Answer from the drawing. Dimensions are ordinates in mm from the lowest x, y and z of the part. A direction names the side the tool comes from. Round coordinates to 2 decimals unless told otherwise and drop trailing zeros. Write each loop counter-clockwise with the first axis right and the second up, starting at its lowest first coordinate (ties: lowest second). Pieces come first, ordered by that corner, then holes. Notation, with made-up numbers: (2.5, 16) - (59.5, 16) arc R16 cw to (59.5, 25) - close; hole circle Ø4 at (20, 40). An arc over 180 degrees is marked (long way). Answer as a JSON object with one key per item and string values.
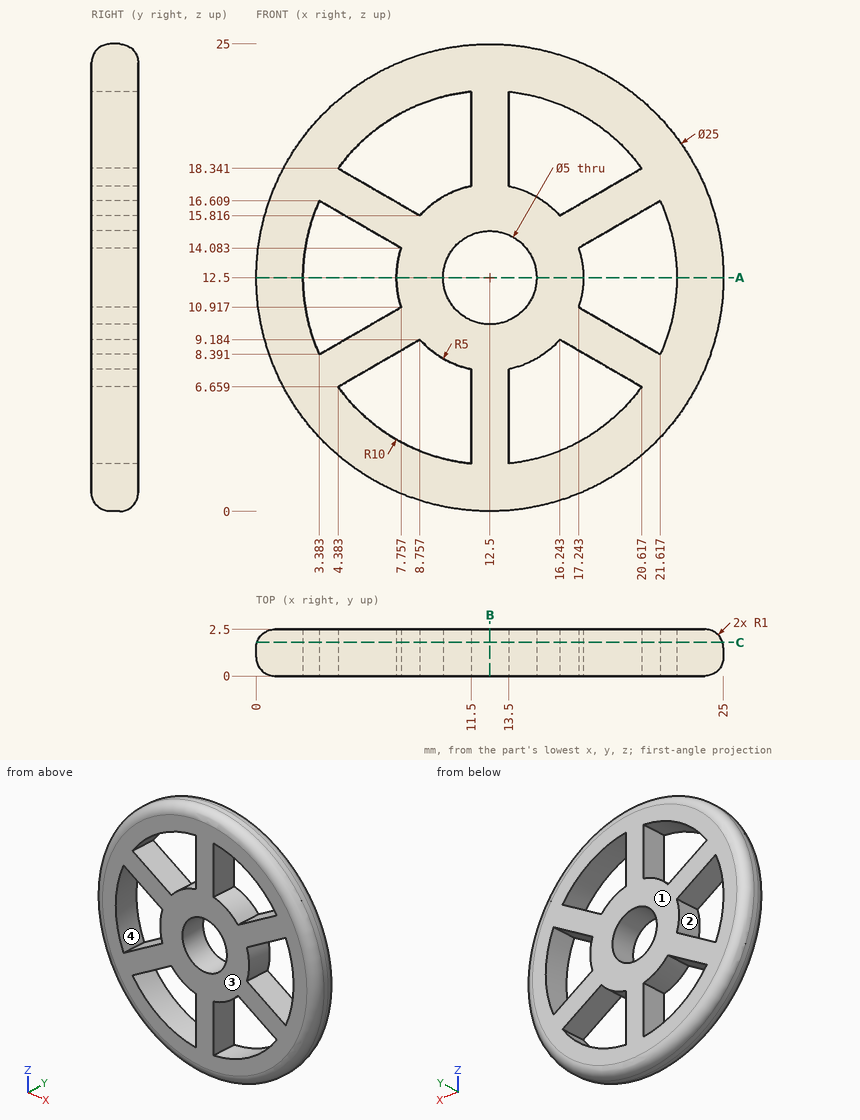
Item 1: A cutting plane is placed at A-A (z = 12.5). Write down the section's boundary in (x, y).
Results found:
{"outline": "(0, 1) arc R1 ccw to (1, 0) - (2.5, 0) - (2.5, 2.5) - (1, 2.5) arc R1 ccw to (0, 1.5) - close; (7.5, 0) - (10, 0) - (10, 2.5) - (7.5, 2.5) - close; (15, 0) - (17.5, 0) - (17.5, 2.5) - (15, 2.5) - close; (22.5, 0) - (24, 0) arc R1 ccw to (25, 1) - (25, 1.5) arc R1 ccw to (24, 2.5) - (22.5, 2.5) - close"}
Item 2: A cutting plane is placed at C-C (y = 1.8). Give the number of separate pieces and of enclosed holes in the cut face, and give its area (3 significant figures).
Results found:
{"separate pieces": "1", "enclosed holes": "7", "area": "292 mm²"}
Item 3: Each of these flat-tipped pins is pushed along its axis until it touches: P1, Ø1, axis at x = 20, y = 1.5, coming from the +Z side (1 decimal); P2, Ø1.2, axis at y = 1, z = 5, coming from the -X side; P3, Ø1.5, axis at x = 21, y = 2, coming from the -Z side (1 decimal). Where does it stop, or does it pass through?
Results found:
{"P1": "z = 22.9", "P2": "x = 2.08", "P3": "z = 2.8"}
Item 4: A cutting plane is placed at B-B (x = 12.5). Write down the section's boundary in (y, z).
Results found:
{"outline": "(0, 1) arc R1 ccw to (1, 0) - (1.5, 0) arc R1 ccw to (2.5, 1) - (2.5, 10) - (0, 10) - close; (0, 15) - (2.5, 15) - (2.5, 24) arc R1 ccw to (1.5, 25) - (1, 25) arc R1 ccw to (0, 24) - close"}
Item 5: Consider line 1 along X through (y, z) = (2, 8.75) (1 decimal); line 2 along Z through (x, y) = (12.5, 1); line 3 along Z through (x, y) = (17.75, 1.15) (1 decimal). Determine where each line is inside the solid, lowest interval first.
Results found:
{"line 1": "0.7 to 3.2, 4 to 8, 9.2 to 15.8, 17 to 21, 21.8 to 24.3", "line 2": "0 to 10, 15 to 25", "line 3": "1.2 to 4, 8.3 to 10.6, 14.4 to 16.7, 21 to 23.8"}
Item 6: Determine the mould class of the marked faces 3 and 4 for opening direction Z: pulls with the +Z half, pulls with the -Z half, needs draft (parallel to the pull), parting line crosses it, or undercut.
Results found:
{"face 3": "needs draft", "face 4": "undercut"}
Item 7: For the marked faces 1 and 2, determine the directions among +Z, -Z, +X, -X, +Y, -Y from which every point of the face is accessible in a straight line to the end or side of a thin tool.
Results found:
{"face 1": "+Z, -Z, +X, -X, +Y", "face 2": "+Y, -Y"}
